from build123d import *

# Parameters (mm, degrees)
EXTRUDE_1_DEPTH     = 55
EXTRUDE_2_DEPTH     = 2
SKETCH_3_R          = 53
EXTRUDE_3_DEPTH     = 3
SKETCH_4_R          = 51.6
CUT_EXTRUDE_1_DEPTH = 2
SKETCH_5_R          = 41
CUT_EXTRUDE_2_DEPTH = 106.220007603
EXTRUDE_START       = 2
SKETCH_6_R          = 42.1
SKETCH_6_R_2        = 41
EXTRUDE_4_DEPTH     = 2
SKETCH_9_W          = 24
SKETCH_9_H          = 47
EXTRUDE_6_DEPTH     = 9
SKETCH_10_W         = 24
SKETCH_10_H         = 37
CUT_EXTRUDE_6_DEPTH = 6
SKETCH_7_R          = 1.1
CUT_EXTRUDE_3_DEPTH = 106.220007603
FILLET_1_R          = 10
CUT_EXTRUDE_7_REACH = 105.683
SKETCH_11_R         = 1.3
FILLET_2_R          = 4.5


with BuildPart() as part:
    # 스케치1 → 보스-돌출1 (new body)
    with BuildSketch(Plane(origin=(0, 0, 0), x_dir=(1, 0, 0), z_dir=(0, 1, 0))):
        Polygon((-68, -47.70428689), (35.844478487, -58.5), (68, -58.5), (68, 58.5), (35.844478487, 58.5), (-68, 47.70428689), align=None)
        Polygon((-65, -45), (36, -55.5), (65, -55.5), (65, 55.5), (36, 55.5), (-65, 45), align=None, mode=Mode.SUBTRACT)
    extrude(amount=EXTRUDE_1_DEPTH)

    # 스케치2 → 보스-돌출2 (add)
    with BuildSketch(Plane(origin=(0, 55, 0), x_dir=(1, 0, 0), z_dir=(0, 1, 0))):
        Polygon((-68, 47.70428689), (35.844478487, 58.5), (68, 58.5), (68, -58.5), (35.844478487, -58.5), (-68, -47.70428689), align=None)
    extrude(amount=EXTRUDE_2_DEPTH)

    # 스케치3 → 보스-돌출3 (add)
    with BuildSketch(Plane.XZ.offset(-55)):
        Circle(SKETCH_3_R)
    extrude(amount=EXTRUDE_3_DEPTH)

    # 스케치4 → 컷-돌출1 (cut)
    with BuildSketch(Plane(origin=(0, 57, 0), x_dir=(1, 0, 0), z_dir=(0, 1, 0))):
        with Locations(Location((0, 0, 0), (0, 0, 270))):
            Circle(SKETCH_4_R)
    extrude(amount=-CUT_EXTRUDE_1_DEPTH, mode=Mode.SUBTRACT)

    # 스케치5 → 컷-돌출2 (cut, through all)
    with BuildSketch(Plane(origin=(0, 55, 0), x_dir=(1, 0, 0), z_dir=(0, 1, 0))):
        with Locations(Location((0, 0, 0), (0, 0, 270))):
            Circle(SKETCH_5_R)
    extrude(amount=-CUT_EXTRUDE_2_DEPTH, mode=Mode.SUBTRACT)

    # 스케치6 → 보스-돌출4 (add)
    with BuildSketch(Plane(origin=(0, 55, 0), x_dir=(1, 0, 0), z_dir=(0, 1, 0)).offset(EXTRUDE_START)):
        with Locations(Location((0, 0, 0), (0, 0, 270))):
            Circle(SKETCH_6_R)
        with Locations(Location((0, 0, 0), (0, 0, 270))):
            Circle(SKETCH_6_R_2, mode=Mode.SUBTRACT)
    extrude(amount=-EXTRUDE_4_DEPTH)

    # 스케치9 → 보스-돌출6 (add)
    with BuildSketch(Plane.XZ.offset(-55)):
        with Locations((53, 0)):
            Rectangle(SKETCH_9_W, SKETCH_9_H)
    extrude(amount=EXTRUDE_6_DEPTH)

    # 스케치10 → 컷-돌출6 (cut)
    with BuildSketch(Plane.XZ.offset(-46)):
        with Locations((53, 0)):
            Rectangle(SKETCH_10_W, SKETCH_10_H)
    extrude(amount=-CUT_EXTRUDE_6_DEPTH, mode=Mode.SUBTRACT)

    # 스케치7 → 컷-돌출3 (cut, through all)
    with BuildSketch(Plane(origin=(0, 55, 0), x_dir=(1, 0, 0), z_dir=(0, 1, 0))):
        with Locations(Location((0, 47.1, 0), (0, 0, 270))):
            Circle(SKETCH_7_R)
        with Locations(Location((27.684685383, 38.104700435, 0), (0, 0, 270))):
            Circle(SKETCH_7_R)
        with Locations(Location((44.794761918, 14.554700435, 0), (0, 0, 270))):
            Circle(SKETCH_7_R)
        with Locations(Location((44.794761918, -14.554700435, 0), (0, 0, 270))):
            Circle(SKETCH_7_R)
        with Locations(Location((27.684685383, -38.104700435, 0), (0, 0, 270))):
            Circle(SKETCH_7_R)
        with Locations(Location((0, -47.1, 0), (0, 0, 270))):
            Circle(SKETCH_7_R)
        with Locations(Location((-27.684685383, -38.104700435, 0), (0, 0, 270))):
            Circle(SKETCH_7_R)
        with Locations(Location((-44.794761918, -14.554700435, 0), (0, 0, 270))):
            Circle(SKETCH_7_R)
        with Locations(Location((-44.794761918, 14.554700435, 0), (0, 0, 270))):
            Circle(SKETCH_7_R)
        with Locations(Location((-27.684685383, 38.104700435, 0), (0, 0, 270))):
            Circle(SKETCH_7_R)
    extrude(amount=-CUT_EXTRUDE_3_DEPTH, mode=Mode.SUBTRACT)

    # 필렛1
    fillet_1_edges = [part.edges().sort_by_distance(p)[0] for p in [
        (-68, 28.5, -47.70428689),
        (68, 28.5, -58.5),
        (68, 28.5, 58.5),
        (-68, 28.5, 47.70428689),
        (-65, 27.5, -45),
        (-65, 27.5, 45),
        (65, 27.5, 55.5),
        (65, 27.5, -55.5),
    ]]
    fillet(fillet_1_edges, radius=FILLET_1_R)

    # 스케치11 → 컷-돌출7 (cut, up to next)
    with BuildSketch(Plane.XZ.offset(-52), mode=Mode.PRIVATE) as cut_extrude_7_sk1:
        with Locations(Location((52, 15.5, 0), (0, 0, 270))):
            Circle(SKETCH_11_R)
    cut_extrude_7_tool1 = extrude(cut_extrude_7_sk1.sketch, amount=-CUT_EXTRUDE_7_REACH, mode=Mode.PRIVATE) & part.part
    # 스케치11 → 컷-돌출7 (cut, up to next)
    with BuildSketch(Plane.XZ.offset(-52), mode=Mode.PRIVATE) as cut_extrude_7_sk2:
        with Locations(Location((52, -15.5, 0), (0, 0, 270))):
            Circle(SKETCH_11_R)
    cut_extrude_7_tool2 = extrude(cut_extrude_7_sk2.sketch, amount=-CUT_EXTRUDE_7_REACH, mode=Mode.PRIVATE) & part.part
    # 스케치11 → 컷-돌출7 (cut, up to next)
    with BuildSketch(Plane.XZ.offset(-52), mode=Mode.PRIVATE) as cut_extrude_7_sk3:
        with Locations(Location((62, 15.5, 0), (0, 0, 270))):
            Circle(SKETCH_11_R)
    cut_extrude_7_tool3 = extrude(cut_extrude_7_sk3.sketch, amount=-CUT_EXTRUDE_7_REACH, mode=Mode.PRIVATE) & part.part
    # 스케치11 → 컷-돌출7 (cut, up to next)
    with BuildSketch(Plane.XZ.offset(-52), mode=Mode.PRIVATE) as cut_extrude_7_sk4:
        with Locations(Location((62, -15.5, 0), (0, 0, 270))):
            Circle(SKETCH_11_R)
    cut_extrude_7_tool4 = extrude(cut_extrude_7_sk4.sketch, amount=-CUT_EXTRUDE_7_REACH, mode=Mode.PRIVATE) & part.part
    add(cut_extrude_7_tool1.solids().sort_by_distance((52, 52, 15.5))[0], mode=Mode.SUBTRACT)
    add(cut_extrude_7_tool2.solids().sort_by_distance((52, 52, -15.5))[0], mode=Mode.SUBTRACT)
    add(cut_extrude_7_tool3.solids().sort_by_distance((62, 52, 15.5))[0], mode=Mode.SUBTRACT)
    add(cut_extrude_7_tool4.solids().sort_by_distance((62, 52, -15.5))[0], mode=Mode.SUBTRACT)

    # 필렛2
    fillet_2_edges = [part.edges().sort_by_distance(p)[0] for p in [
        (53, 46, 23.5),
        (53, 46, -23.5),
        (56.252631433, 55, -23.5),
        (56.252631433, 55, 23.5),
    ]]
    fillet(fillet_2_edges, radius=FILLET_2_R - 0.0001)  # a hair under: the kernel refuses the full size


solid = part.part
Geometry check sheet. Reference: the model listing, model coordinates, mm. A direction names the side the tool comes from. Give positions to 0.01 mm unless a question says otherwise; leave off trailing zeros. Order: outer loops, then holes, each group sorted by start corner. A loop starts at its lowest first (then second) coordinate and runs counter-clockwise, first axis right, second up.
1) Cross-section at B-B (y = 14.5). Record the boundary of the cut face in (x, z).
Results are:
outline: (-68, -38.69) arc R10 ccw to (-59.03, -48.64) - (35.84, -58.5) - (58, -58.5) arc R10 ccw to (68, -48.5) - (68, 48.5) arc R10 ccw to (58, 58.5) - (35.84, 58.5) - (-59.03, 48.64) arc R10 ccw to (-68, 38.69) - close; hole (-65, -35.99) arc R10 ccw to (-56.03, -45.93) - (36, -55.5) - (55, -55.5) arc R10 ccw to (65, -45.5) - (65, 45.5) arc R10 ccw to (55, 55.5) - (36, 55.5) - (-56.03, 45.93) arc R10 ccw to (-65, 35.99) - close
2) Material ranges on probe 1 along Z at (x, y) = (44, 51); probe 2 along X at (y, z) = (4, 8); probe 3 along Z at (x, y) = (37, 24), recorded low to high.
Results are:
probe 1: z = -58.5 to -55.5, -23.53 to -18.5, 18.5 to 23.53, 55.5 to 58.5
probe 2: x = -68 to -65, 65 to 68
probe 3: z = -58.5 to -55.5, 55.5 to 58.5
3) Cross-section at D-D (x = -19.5). Record the boundary of the cut face in (y, z).
Results are:
outline: (0, -52.75) - (57, -52.75) - (57, -47.77) - (55, -47.77) - (55, -37.31) - (57, -37.31) - (57, -36.07) - (52, -36.07) - (52, -49.28) - (55, -49.28) - (55, -49.73) - (0, -49.73) - close; (0, 49.73) - (55, 49.73) - (55, 49.28) - (52, 49.28) - (52, 36.07) - (57, 36.07) - (57, 37.31) - (55, 37.31) - (55, 47.77) - (57, 47.77) - (57, 52.75) - (0, 52.75) - close
4) Cross-section at C-C (x = 30.5). Record the boundary of the cut face in (y, z).
Results are:
outline: (0, -57.94) - (57, -57.94) - (57, -41.62) - (55, -41.62) - (55, -29.02) - (57, -29.02) - (57, -27.4) - (52, -27.4) - (52, -43.34) - (55, -43.34) - (55, -54.93) - (0, -54.93) - close; (0, 54.93) - (55, 54.93) - (55, 43.34) - (52, 43.34) - (52, 27.4) - (57, 27.4) - (57, 29.02) - (55, 29.02) - (55, 41.62) - (57, 41.62) - (57, 57.94) - (0, 57.94) - close
5) Tool access check on faces 1 (the cylindrical face through (55.835, 53.647, -24.783)), 2 (the flat face through (68, 28, -1)). Record the directions out of +Z, -Z, +X, -X, +Y, -Y that give a thin tool (end or side, any length) a straight path to the whole face; none if there is none.
Results are:
face 1: -Y
face 2: +Z, -Z, +X, +Y, -Y
6) Cross-section at A-A (z = -6). Record the boundary of the cut face in (x, y), then the cut area to 3 significant figures.
Results are:
outline: (-68, 0) - (-65, 0) - (-65, 55) - (-52.66, 55) - (-52.66, 52) - (-40.56, 52) - (-40.56, 57) - (-41.67, 57) - (-41.67, 55) - (-51.25, 55) - (-51.25, 57) - (-68, 57) - close; (40.56, 52) - (65, 52) - (65, 0) - (68, 0) - (68, 57) - (51.25, 57) - (51.25, 55) - (41.67, 55) - (41.67, 57) - (40.56, 57) - close
area: 511 mm2
7) Draft check along Z on faces 3 (the flat face through (-10.931, 28.101, 53.637)), 4 (the flat face through (53, 49, 18.5)), 5 (the flat face through (-40.3, 57, 9.2)). Enter one of: released by +Z, released by -Z, zero draft, split by the parting line, or undercut.
Results are:
face 3: released by +Z
face 4: undercut
face 5: zero draft
8) Gauge pin test, flat ends, axial feed: pin 1 (3 mm diameter, centred on x = -44.79, z = 14.55, fed in from -Y); pin 2 (3 mm diameter, centred on x = -27.68, z = -38.1, fed in from +Y); pin 3 (1.5 mm diameter, centred on x = -14, y = 7.5, fed in from -Z). Record the tip position at first contact, or that the pin passes through.
Results are:
pin 1: stops at y = 52
pin 2: stops at y = 55
pin 3: stops at z = -53.4
